The listing builds one solid part. Answer for the finished solid, in the listing's coordinates (mm). A direction names the side the tool comes from. Give positions to 0.01 mm unless a question says otherwise; leave off trailing zeros. Loops run counter-clockwise (first coordinate to the right, second up) from the corner with the lowest first, then second, coordinate; pieces in that order, holes last. Notation, with made-up numbers: (-7, -27) - (28, -27) arc R14 cw to (28, -10) - close; hole circle Ø6 at (22, 57). An arc over 180 degrees is marked (long way). Write each question's results on one line, items separated by ' | '.
from build123d import *

# Parameters (mm, degrees)
F2_R     = 4.699
F3_DEPTH = 9.525
F4_R     = 1.5875
F5_DEPTH = 12.7


with BuildPart() as f1:
    # F0 (on Front) → F1 (revolve)
    with BuildSketch(Plane.XZ):
        with BuildLine():
            Line((0, 50.8), (0, 0))
            Line((0, 0), (3.81, 0))
            Line((3.81, 0), (10.16, 6.35))
            Line((10.16, 6.35), (19.05, 6.35))
            Line((19.05, 6.35), (19.05, 5.08))
            ThreePointArc((19.05, 5.08), (20.165923, 2.385923), (22.86, 1.27))
            Line((22.86, 1.27), (25.4, 1.27))
            ThreePointArc((25.4, 1.27), (28.094077, 2.385923), (29.21, 5.08))
            Line((29.21, 5.08), (29.21, 13.97))
            ThreePointArc((29.21, 13.97), (28.094077, 16.664077), (25.4, 17.78))
            Line((25.4, 17.78), (22.86, 17.78))
            ThreePointArc((22.86, 17.78), (20.165923, 16.664077), (19.05, 13.97))
            Line((19.05, 13.97), (19.05, 12.7))
            Line((19.05, 12.7), (10.16, 12.7))
            Line((10.16, 12.7), (10.16, 50.8))
            Line((10.16, 50.8), (0, 50.8))
        make_face()
    revolve(axis=Axis((0, 0, 25.4), (0, 0, -1)))

    # F2 (on face) → F3 (cut)
    with BuildSketch(Plane.XY.offset(50.8)):
        Circle(F2_R)
    extrude(amount=-F3_DEPTH, mode=Mode.SUBTRACT)

    # F4 (on face) → F5 (cut)
    with BuildSketch(Plane(origin=(0, 0, 0), x_dir=(1, 0, 0), z_dir=(0, 0, -1))):
        Circle(F4_R)
    extrude(amount=-F5_DEPTH, mode=Mode.SUBTRACT)


solid = f1.part
Item 1: A cutting plane is placed at A-A, the plane z = 8.5. Determine the outline of the cut face in (x, y) (1 decimal).
Values found:
outline: circle Ø58.4 at (0, 0); hole circle Ø3.2 at (0, 0)
Item 2: Find the intervals of material crossed by line 1 along X through (y, z) = (0, 13.15); line 2 along X through (y, z) = (-2.5, 2), in increasing order. Write a range as [from, to].
Values found:
line 1: x = [-29.21, -19.05], [-10.16, 10.16], [19.05, 29.21] | line 2: x = [-27.53, -20.47], [-5.24, 5.24], [20.47, 27.53]
Item 3: A cutting plane is placed at B-B, the plane z = 17. Determine the outline of the cut face in (x, y).
Values found:
outline: circle Ø55.42 at (0, 0); circle Ø20.32 at (0, 0); hole circle Ø41.1 at (0, 0)
Item 4: A cutting plane is placed at C-C, the plane z = 43.5. Determine the outline of the cut face in (x, y).
Values found:
outline: circle Ø20.32 at (0, 0); hole circle Ø9.4 at (0, 0)
Item 5: For faces 1 (the face through (8, 8, 12.7)), 2 (the face through (-15.12, 11.59, 5.71)), 3 (the face through (2.1, 4.4, 50.8)), determine the directions among +Z, -Z, +X, -X, +Y, -Y from which every point of the face is accessible in a straight line to the end or side of a thin tool.
Values found:
face 1: +Z | face 2: -Z | face 3: +Z, +X, -X, +Y, -Y
Item 6: Flat-ended cylindrical pins translate along their axes: P1, Ø6, axis at x = 4.5, y = -8, coming from the -Z side; P2, Ø6, axis at x = -5.5, z = 36, coming from the +Y side; P3, Ø4, axis at x = 0, z = 23.5, coming from the -Y side. Find the tip coordinate at first contact, or state that the pin passes through.
Values found:
P1: stops at z = 2.37 | P2: stops at y = 9.85 | P3: stops at y = -10.16
Item 7: For a pull along X with two mould halves and no side action, classify faces 4 (the face through (0, 0, 12.7)), 5 (the face through (0, 2, 0)), 6 (the face through (-21.53, -19.74, 9.59)) as released by +X, released by -X, zero draft, split by the parting line, or undercut.
Values found:
face 4: undercut | face 5: zero draft | face 6: split by the parting line
